Could you check a few things on this model? Use its own coordinates, in mm. Face numbers are marked on the shaded views. A direction names the side the tool comes from. Give positions to 0.01 mm unless a question says otherwise; leave off trailing zeros. Order: outer loops, then holes, each group sorted by start corner. A loop starts at its lowest first (then second) coordinate and runs counter-clockwise, first axis right, second up.
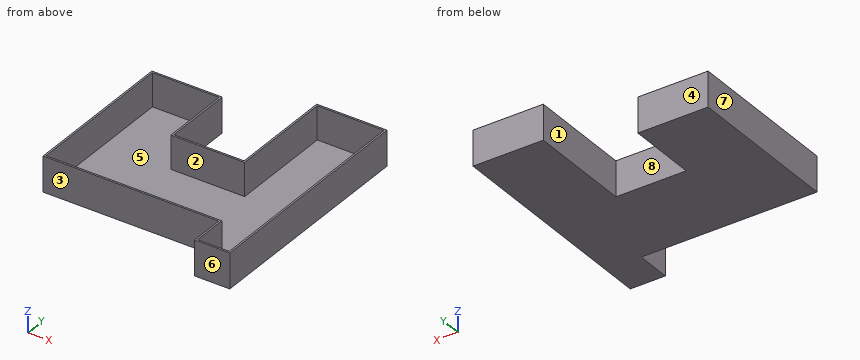
Autodesk Inventor part; units mm, degrees
ref_plane "YZ Plane" through (0, 0, 0) normal (1, 0, 0) x (0, 1, 0)
ref_plane "XZ Plane" through (0, 0, 0) normal (0, 1, 0) x (-1, 0, 0)
ref_plane "XY Plane" through (0, 0, 0) normal (0, 0, 1) x (1, 0, 0)
sketch "Sketch1" plane through (0, 0, 0) normal (0, 0, 1) x (1, 0, 0)
  line L0 (0, 2.4004) -> (60, 2.4004) construction
  line L1 (-60, 0) -> (60, 0) construction
  line L2 (-60, 0) -> (-60, 20) construction
  line L3 (-60, 20) -> (40, 20)
  line L4 (40, 20) -> (40, 0)
  line L5 (40, 0) -> (60, 0)
  line L6 (60, 0) -> (60, 130)
  line L7 (75, 0) -> (75, 70) construction
  line L8 (-60, 20) -> (-60, 110)
  line L9 (-60, 110) -> (-20, 110)
  line L10 (-20, 110) -> (-20, 70)
  line L11 (-20, 70) -> (20, 70)
  line L12 (20, 70) -> (20, 130)
  line L13 (20, 130) -> (60, 130)
  point P0 (0, 0)
  dimension "d2" = 120
  dimension "d3" = 20
  dimension "d4" = 100
  dimension "d5" = 20
  dimension "d6" = 20
  dimension "d7" = 130
  dimension "d8" = 70
  dimension "d9" = 90
  dimension "d10" = 40
  dimension "d11" = 40
extrude "Extrusion1" add sketch "Sketch1" along normal blind 20
shell "Shell1" thickness 1 removed faces 1 at (-13.3333, 36.6667, 20)
properties part number "Spacer_3DPrint"
Item 1: We'd pull the mould along Y, two halves only. Please class the marked faces 5, 6, 7 and 8: +Y half, -Y half, draft (parallel to the pull), parting line (faces both ways), or undercut.
Findings:
face 5: undercut
face 6: -Y half
face 7: draft
face 8: +Y half
Item 2: Please list where these lines run through material, in increasing order: line 1 along X through (y, z) = (91.5, 9.5); line 2 along Y through (x, z) = (17.5, 3.5); line 3 along X through (y, z) = (46, 3).
Findings:
line 1: x = -60 to -59, -21 to -20, 20 to 21, 59 to 60
line 2: y = 20 to 21, 69 to 70
line 3: x = -60 to -59, 59 to 60
Item 3: For pin 1 (1 mm diameter, centred on x = 3.5, z = 2.5, fed in from +Y); pin 2 (6 mm diameter, centred on x = 14.5, z = 9, fed in from -Y); pin 3 (10 mm diameter, centred on x = -30, z = 8, fed in from +Y); pin 4 (8 mm diameter, centred on x = 47.5, z = 10.5, fed in from -Y), each with a flat end and sliding along its axis, tell me the tip position at first contact or that it passes through.
Findings:
pin 1: stops at y = 70
pin 2: stops at y = 20
pin 3: stops at y = 110
pin 4: stops at y = 0
Item 4: Imagine slicing it at D-D on y = 27. List the corners of the cut face in (x, z) for me, then the cut area to 3 significant figures.
Findings:
outline: (-60, 0) - (60, 0) - (60, 20) - (59, 20) - (59, 1) - (-59, 1) - (-59, 20) - (-60, 20) - close
area: 158 mm2
Item 5: For the marked faces 1, 2, 3 and 4, which set-ups out of +Z, -Z, +X, -X, +Y, -Y let a thin tool reach every point of the face, with its end or its side?
Findings:
face 1: +Z, -Z, +Y
face 2: +Z
face 3: +Z, -Z, -X, -Y
face 4: +Z, -Z, -X, +Y
Item 6: Imagine slicing it at B-B on y = 100. List the corners of the cut face in (x, z) for me, then the cut area to 3 significant figures.
Findings:
outline: (-60, 0) - (-20, 0) - (-20, 20) - (-21, 20) - (-21, 1) - (-59, 1) - (-59, 20) - (-60, 20) - close; (20, 0) - (60, 0) - (60, 20) - (59, 20) - (59, 1) - (21, 1) - (21, 20) - (20, 20) - close
area: 156 mm2
Item 7: Imagine slicing it at A-A on z = 18.5. List the corners of the cut face in (x, y) for me.
Findings:
outline: (-60, 20) - (40, 20) - (40, 0) - (60, 0) - (60, 130) - (20, 130) - (20, 70) - (-20, 70) - (-20, 110) - (-60, 110) - close; hole (-59, 21) - (41, 21) - (41, 1) - (59, 1) - (59, 129) - (21, 129) - (21, 69) - (-21, 69) - (-21, 109) - (-59, 109) - close
Item 8: Imagine slicing it at C-C on x = 29. List the corners of the cut face in (y, z) for me.
Findings:
outline: (20, 0) - (130, 0) - (130, 20) - (129, 20) - (129, 1) - (21, 1) - (21, 20) - (20, 20) - close
